from build123d import *

# Parameters (mm, degrees)
F0_R     = 6.9
F1_DEPTH = 40
F3_DEPTH = 40
F4_W     = 11.228349
F4_H     = 10.522324
F5_DEPTH = 3.5
F6_W     = 11.228349
F6_H     = 16.9586
F7_DEPTH = 3.5
F8_R     = 4.547119
F9_DEPTH = 2.5


with BuildPart() as f1:
    # F0 (on Top) → F1 (new body)
    with BuildSketch(Plane.XY):
        with Locations((-26.366409, 6.635255)):
            Circle(F0_R)
    extrude(amount=F1_DEPTH)

    # F2 (on face) → F3 (cut)
    with BuildSketch(Plane(origin=(0, 0, 0), x_dir=(1, 0, 0), z_dir=(0, 0, -1))):
        Polygon((-17.36803, 0.397698), (-23.011649, -0.605696), (-21.749303, -11.76286), (-16.136123, -11.266587), align=None)
    extrude(amount=-F3_DEPTH, mode=Mode.SUBTRACT)

    # F4 (on face) → F5 (join)
    with BuildSketch(Plane(origin=(-22.78846, 2.578335, 0), x_dir=(0.112425, 0.99366, 0), z_dir=(0.99366, -0.112425, 0))):
        with Locations((3.62895, 45.261162)):
            Rectangle(F4_W, F4_H)
    extrude(amount=-F5_DEPTH)

    # F6 (on face) → F7 (join)
    with BuildSketch(Plane(origin=(-22.78846, 2.578335, 0), x_dir=(0.112425, 0.99366, 0), z_dir=(0.99366, -0.112425, 0))):
        with Locations((3.62895, 59.001624)):
            Rectangle(F6_W, F6_H)
    extrude(amount=-F7_DEPTH)

    # F8 (on face) → F9 (cut)
    with BuildSketch(Plane(origin=(-26.266271, 2.971822, 0), x_dir=(-0.112425, -0.99366, 0), z_dir=(-0.99366, 0.112425, 0))):
        with Locations((-3.642559, 59.778914)):
            Circle(F8_R)
    extrude(amount=-F9_DEPTH, mode=Mode.SUBTRACT)


solid = f1.part
Geometry: final body of the model. Coordinates: model frame, mm. A direction names the side the tool comes from. Coordinates: 2 decimals unless noted, no trailing zeros. Loops run counter-clockwise (first coordinate to the right, second up) from the corner with the lowest first, then second, coordinate; pieces in that order, holes last. Notation, with made-up numbers: (-30, -1.75) - (2, -1.75) arc R20 ccw to (2, 18.25) - close; hole circle Ø1 at (-20, -28). An arc over 180 degrees is marked (long way). Put each result on its own line as item: value. Start each with the question number.
Q1. Cut plane D-D, the plane x = -30.5. Return loops of the section in (y, z), and give its area (3 significant figures).
Q2. Pin query (flat end, axial travel): pin 1 Ø6 at (x, y) = (-31, 10) entering from +Z; pin 2 Ø4 at (x, z) = (-23.5, 58.5) entering from +Y; pin 3 Ø3 at (y, z) = (12, 39) entering from -X. Return the tip coordinate at first contact, or that it passes through.
Q3. Pull-direction query (Z, two-part tool) for faces 1 (the flat face through (-24, 6, 67.481)), 2 (the cylindrical face through (-24.566, 7.041, 64.287)), 3 (the flat face through (-25.867, 6.5, 50.879)); classes: released by +Z, released by -Z, zero draft, split by the parting line, or undercut.
Q4. Cut plane B-B, the plane x = -27.75. Return loops of the section in (y, z).
Q5. Cut plane C-C, the plane z = 5. Return loops of the section in (x, y).
Q6. Set-up query: faces 4 (the flat face through (-24.73, 0.8, 53.55)), 5 (the flat face through (-22.39, 6.11, 19.72)), 6 (the flat face through (-23.464, 11.957, 53.548)). Return all of +Z, -Z, +X, -X, +Y, -Y with unobstructed straight access to the full face (end or side cutting, diameter ignored); none if empty.
Q7. Line query: line 1 (Z direction, x = -25.25, y = 8); line 2 (Z direction, x = -29.25, y = 0.75); line 3 (Y direction, x = -26, z = 29) (3 decimals). Output: solid intervals per line, ascending.
Q8. Cut plane A-A, the plane z = 58. Return loops of the section in (x, y), and give its area (3 significant figures).
Filled sheet:
1. outline: (1.11, 0) - (12.16, 0) - (12.16, 40) - (1.11, 40) - close
1. area: 442 mm²
2. pin 1: z = 40
2. pin 2: y = 12.16
2. pin 3: x = -32.08
3. face 1: released by +Z
3. face 2: undercut
3. face 3: zero draft
4. outline: (-0.12, 0) - (13.4, 0) - (13.4, 40) - (-0.12, 40) - close
5. outline: (-23.01, 0.61) - (-21.75, 11.76) arc R6.9 ccw (long way) to start
6. face 4: +Z, -X, -Y
6. face 5: +Z, -Z, +X, -Y
6. face 6: +Z, +X, +Y
7. line 1: 0 to 55.48, 64.08 to 67.48
7. line 2: 0 to 40
7. line 3: -0.255 to 13.526
8. outline: (-26.49, 1) - (-23.01, 0.61) - (-21.75, 11.76) - (-25.23, 12.16) - (-25.39, 10.75) - (-22.9, 10.47) - (-23.84, 2.15) - (-26.33, 2.43) - close
8. area: 18.4 mm²
